Autodesk Inventor part; units mm, degrees
ref_plane "YZ Plane" through (0, 0, 0) normal (1, 0, 0) x (0, 1, 0)
ref_plane "XZ Plane" through (0, 0, 0) normal (0, 1, 0) x (-1, 0, 0)
ref_plane "XY Plane" through (0, 0, 0) normal (0, 0, 1) x (1, 0, 0)
sketch "Sketch1" plane through (0, 0, 0) normal (0, 1, 0) x (-1, 0, 0)
  arc A0 (0, 2.5) -> (0, -2.5) centre (0, 0) ccw
  line L0 (0, -2.5) -> (15, -2.5)
  line L1 (15, -2.5) -> (15, 2.5)
  line L2 (15, 2.5) -> (0, 2.5)
  dimension "d0" = 5
  dimension "d1" = 15
extrude "Extrusion1" add sketch "Sketch1" along normal blind 25
sketch "Sketch2" plane through (-15, 0, 2.5) normal (0, 0, 1) x (1, 0, 0)
  line L0 (0, 0) -> (15, 0) construction
  line L1 (15, 0) -> (15, 25) construction
  line L2 (0, 25) -> (15, 25) construction
  line L3 (0, 0) -> (0, 25) construction
  line L4 (0, 0) -> (0, 25) construction
  line L5 (15, 6.5) -> (0, 6.5) construction
  line L6 (0, 6.5) -> (0, 18.5) construction
  line L7 (0, 18.5) -> (15, 18.5) construction
  line L8 (15, 18.5) -> (15, 6.5) construction
  line L9 (15, 12.5) -> (0, 12.5) construction
  line L10 (15, 6.5) -> (0, 0) construction
  line L11 (15, 0) -> (0, 0) construction
  line L12 (0, 6.5) -> (15, 0) construction
  line L13 (15, 25) -> (0, 25) construction
  line L14 (15, 25) -> (0, 18.5) construction
  line L15 (0, 25) -> (15, 18.5) construction
  line L16 (11.5, 21.75) -> (3.5, 21.75) construction
  line L17 (11.5, 23.35) -> (3.5, 23.35)
  line L18 (3.5, 20.15) -> (11.5, 20.15)
  arc A0 (11.5, 20.15) -> (11.5, 23.35) centre (11.5, 21.75) ccw
  arc A1 (3.5, 23.35) -> (3.5, 20.15) centre (3.5, 21.75) ccw
  line L19 (11.5, 3.25) -> (3.5, 3.25) construction
  line L20 (11.5, 1.65) -> (3.5, 1.65)
  line L21 (3.5, 4.85) -> (11.5, 4.85)
  arc A2 (11.5, 1.65) -> (11.5, 4.85) centre (11.5, 3.25) ccw
  arc A3 (3.5, 4.85) -> (3.5, 1.65) centre (3.5, 3.25) ccw
  point P0 (7.5, 21.75)
  point P1 (7.5, 21.75)
  point P2 (7.5, 3.25)
  point P3 (7.5, 3.25)
  dimension "d4" = 12
  dimension "d5" = 3.2
  dimension "d6" = 8
extrude "Extrusion2" cut sketch "Sketch2" against normal through all
ref_plane "Work Plane2" through (-15, 12.5, 2.5) normal (0, 1, 0) x (1, 0, 0)
fillet "Fillet1" radius 2.5 2 edges at (-15, 0, 0) (-15, 25, 0)
properties part number "FixedClamp"
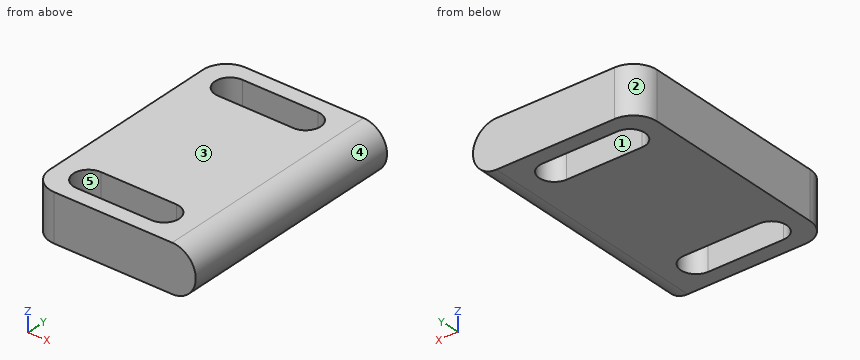
Read the model definition and answer for the solid it produces. Units are mm, in the model's axes. Face numbers are marked on the shaded views. A direction names the side the tool comes from. Coordinates: 2 decimals unless noted, no trailing zeros. Loops run counter-clockwise (first coordinate to the right, second up) from the corner with the lowest first, then second, coordinate; pieces in that order, holes last. Notation, with made-up numbers: (21, 44) - (50, 44) arc R28 ccw to (50, 66) - close; hole circle Ø8 at (-24, -14.5). An arc over 180 degrees is marked (long way). Answer in a Markdown table with one row per item.
Q1. For the marked faces 1 and 2, determine the directions among +Z, -Z, +X, -X, +Y, -Y from which every point of the face is accessible in a straight line to the end or side of a thin tool.
Here are the results:
| item | result |
|---|---|
| face 1 | +Z, -Z |
| face 2 | +Z, -Z, -X, +Y |
Q2. The mould has two halves that part along X. Classify the marked faces 3, 4 and 5: pulls with the +X half, pulls with the -X half, needs draft (parallel to the pull), parting line crosses it, or undercut.
Here are the results:
| item | result |
|---|---|
| face 3 | needs draft |
| face 4 | pulls with the +X half |
| face 5 | undercut |
Q3. Find section A-A on y = 3.25. Write down the section's boundary in (x, z).
Here are the results:
| item | result |
|---|---|
| outline | (-15, -2.5) - (-13.1, -2.5) - (-13.1, 2.5) - (-15, 2.5) - close; (-1.9, -2.5) - (0, -2.5) arc R2.5 ccw to (0, 2.5) - (-1.9, 2.5) - close |
Q4. Find section C-C on z = 0. Write down the section's boundary in (x, y).
Here are the results:
| item | result |
|---|---|
| outline | (-15, 2.5) arc R2.5 ccw to (-12.5, 0) - (2.5, 0) - (2.5, 25) - (-12.5, 25) arc R2.5 ccw to (-15, 22.5) - close; hole (-11.5, 1.65) - (-3.5, 1.65) arc R1.6 ccw to (-3.5, 4.85) - (-11.5, 4.85) arc R1.6 ccw to start; hole (-11.5, 20.15) - (-3.5, 20.15) arc R1.6 ccw to (-3.5, 23.35) - (-11.5, 23.35) arc R1.6 ccw to start |
Q5. Find section D-D on z = 1.4. Write down the section's boundary in (x, y).
Here are the results:
| item | result |
|---|---|
| outline | (-15, 2.5) arc R2.5 ccw to (-12.5, 0) - (2.07, 0) - (2.07, 25) - (-12.5, 25) arc R2.5 ccw to (-15, 22.5) - close; hole (-11.5, 1.65) - (-3.5, 1.65) arc R1.6 ccw to (-3.5, 4.85) - (-11.5, 4.85) arc R1.6 ccw to start; hole (-11.5, 20.15) - (-3.5, 20.15) arc R1.6 ccw to (-3.5, 23.35) - (-11.5, 23.35) arc R1.6 ccw to start |
Q6. Straight lines are drawn through the part: line 1 along Y through (x, z) = (-9, 1.1); line 2 along Y through (x, z) = (-2.5, 1.15); line 3 along X through (y, z) = (13.25, 1.3). For each, find the intervals that lie inside material, in ascending order. Write a range as [from, to].
Here are the results:
| item | result |
|---|---|
| line 1 | y = [0, 1.65], [4.85, 20.15], [23.35, 25] |
| line 2 | y = [0, 2], [4.5, 20.5], [23, 25] |
| line 3 | x = [-15, 2.14] |
Q7. Find section B-B on x = -8.5. Write down the section's boundary in (y, z).
Here are the results:
| item | result |
|---|---|
| outline | (0, -2.5) - (1.65, -2.5) - (1.65, 2.5) - (0, 2.5) - close; (4.85, -2.5) - (20.15, -2.5) - (20.15, 2.5) - (4.85, 2.5) - close; (23.35, -2.5) - (25, -2.5) - (25, 2.5) - (23.35, 2.5) - close |
